Input: dimensioned drawing with shaded views. Units: mm. Origin: part minimum x, y, z. Round coordinates to 2 decimals unless told otherwise and drop trailing zeros. Loops run counter-clockwise (first coordinate to the right, second up) from the corner with the lowest first, then second, coordinate; pieces in that order, holes last.
1) Section B-B, the plane y = 32.25. Return loops of the section in (x, z), and give its area (4 significant figures).
2) Section D-D, the plane x = 19.25. Return loops of the section in (y, z).
3) Ray query, line 1 along Y through (x, z) = (19.25, 1.65); line 2 along X through (y, z) = (9, 2); line 3 along Y through (x, z) = (18, 2.8). Return the intervals inside material, ascending.
4) First-contact query: pin 1 (10 mm diameter, centred on x = 33, y = 8, fed in from +Z); pin 2 (2 mm diameter, centred on x = 4.5, y = 12.5, fed in from +Z); pin 3 (1.6 mm diameter, centred on y = 10.5, z = 2, fed in from +X); pin 4 (1.5 mm diameter, centred on y = 13.5, z = 1, fed in from -X). Flat tips, straight axial feed; report the tip coordinate or a pass-through.
5) Section A-A, the plane x = 15. Return loops of the section in (y, z), and give its area (3 significant figures).
6) Section C-C, the plane z = 2.35. Return loops of the section in (x, y).
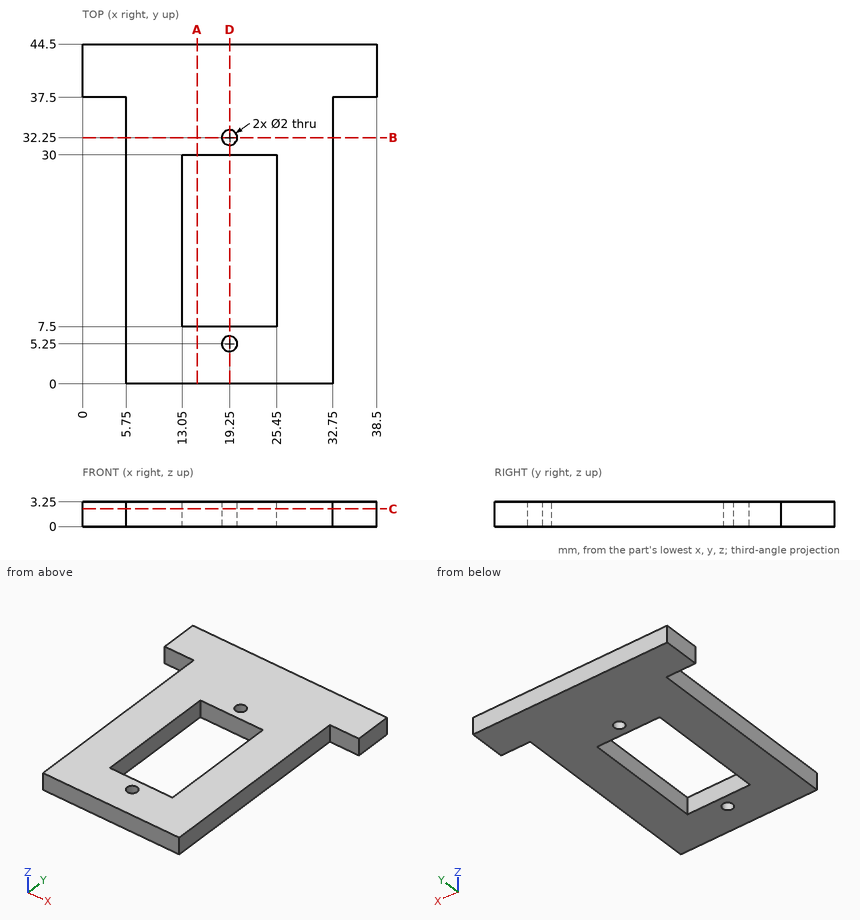
Final values:
1. outline: (5.75, 0) - (18.25, 0) - (18.25, 3.25) - (5.75, 3.25) - close; (20.25, 0) - (32.75, 0) - (32.75, 3.25) - (20.25, 3.25) - close
1. area: 81.25 mm2
2. outline: (0, 0) - (4.25, 0) - (4.25, 3.25) - (0, 3.25) - close; (6.25, 0) - (7.5, 0) - (7.5, 3.25) - (6.25, 3.25) - close; (30, 0) - (31.25, 0) - (31.25, 3.25) - (30, 3.25) - close; (33.25, 0) - (44.5, 0) - (44.5, 3.25) - (33.25, 3.25) - close
3. line 1: y = 0 to 4.25, 6.25 to 7.5, 30 to 31.25, 33.25 to 44.5
3. line 2: x = 5.75 to 13.05, 25.45 to 32.75
3. line 3: y = 0 to 7.5, 30 to 44.5
4. pin 1: stops at z = 3.25
4. pin 2: passes through
4. pin 3: stops at x = 32.75
4. pin 4: stops at x = 5.75
5. outline: (0, 0) - (7.5, 0) - (7.5, 3.25) - (0, 3.25) - close; (30, 0) - (44.5, 0) - (44.5, 3.25) - (30, 3.25) - close
5. area: 71.5 mm2
6. outline: (0, 37.5) - (5.75, 37.5) - (5.75, 0) - (32.75, 0) - (32.75, 37.5) - (38.5, 37.5) - (38.5, 44.5) - (0, 44.5) - close; hole (13.05, 7.5) - (25.45, 7.5) - (25.45, 30) - (13.05, 30) - close; hole circle Ø2 at (19.25, 5.25); hole circle Ø2 at (19.25, 32.25)
